Input: part model. Units: mm. Frame: model coordinates. Face numbers are marked on the shaded views. A direction names the side the tool comes from. Coordinates: 2 decimals unless noted, no trailing zeros. Write each loop counter-clockwise with the first axis right and the second up, starting at its lowest first coordinate (ties: lowest second). Pieces come first, ordered by that corner, then holes.
1) Section query A-A (y = 8). Output: boundary loops of the cut face in (x, z), then the cut area to 3 significant figures.
2) Section query B-B (z = 3.75). Output: boundary loops of the cut face in (x, y), then the cut area to 3 significant figures.
3) Pin query (flat end, axial travel): pin 1 Ø1.5 at (x, z) = (-2.5, 3.5) entering from -Y; pin 2 Ø0.7 at (x, y) = (5, 0) entering from +Z; pin 3 Ø3.5 at (x, z) = (-3.5, 2.5) entering from +Y; pin 4 Ø8 at (x, y) = (-16.5, 3) entering from -Z. Return the tip coordinate at first contact, or that it passes through.
4) Section query C-C (y = 0). Output: boundary loops of the cut face in (x, z), then the cut area to 3 significant figures.
5) Set-up query: the marked faces 1, 2 and 3. Return all of +Z, -Z, +X, -X, +Y, -Y with unobstructed straight access to the full face (end or side cutting, diameter ignored); none if empty.
6) Line query: L1, parallel to X at y = 4.75, z = -1; L2, parallel to Y at x = -33, z = 3.75; L3, parallel to Z at x = -10, y = -0.25. Output: solid intervals per line, ascending.
7) Section query D-D (x = -31). Output: boundary loops of the cut face in (y, z), then the cut area to 3 significant figures.
from build123d import *

# Parameters (mm, degrees)
SKETCH1_W           = 70
SKETCH1_H           = 5
SKETCH1_W_2         = 67
SKETCH1_H_2         = 1.4
BOSS_EXTRUDE1_DEPTH = 5
SKETCH2_W           = 70
SKETCH2_H           = 5
BOSS_EXTRUDE2_DEPTH = 2
BOSS_EXTRUDE3_DEPTH = 2.5
BOSS_EXTRUDE4_DEPTH = 2.5


with BuildPart() as part:
    # Sketch1 → Boss-Extrude1 (new body)
    with BuildSketch(Plane.XY):
        Rectangle(SKETCH1_W, SKETCH1_H)
        Rectangle(SKETCH1_W_2, SKETCH1_H_2, mode=Mode.SUBTRACT)
    extrude(amount=BOSS_EXTRUDE1_DEPTH)

    # Sketch2 → Boss-Extrude2 (add)
    with BuildSketch(Plane(origin=(0, 0, 0), x_dir=(-1, 0, 0), z_dir=(0, 0, -1))):
        Rectangle(SKETCH2_W, SKETCH2_H)
    extrude(amount=BOSS_EXTRUDE2_DEPTH)

    # Sketch3 → Boss-Extrude3 (add)
    with BuildSketch(Plane(origin=(35, 0, 0), x_dir=(0, 0, -1), z_dir=(1, 0, 0))):
        Polygon((-5, 2.5), (2, 15), (2, -15), (-5, -2.5), align=None)
    extrude(amount=BOSS_EXTRUDE3_DEPTH)

    # Sketch4 → Boss-Extrude4 (add)
    with BuildSketch(Plane.ZY.offset(35)):
        Polygon((5, 2.5), (-2, 15), (-2, -15), (5, -2.5), align=None)
    extrude(amount=BOSS_EXTRUDE4_DEPTH)


solid = part.part
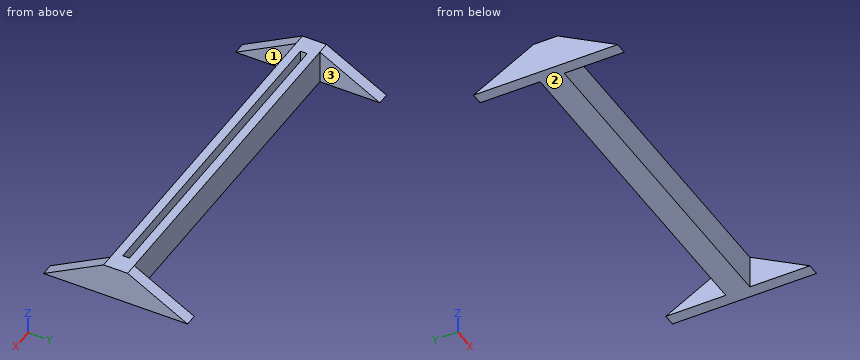
Answer:
1. outline: (-37.5, -2) - (-35, -2) - (-35, 1.92) - (-37.5, 1.92) - close; (35, -2) - (37.5, -2) - (37.5, 1.92) - (35, 1.92) - close
1. area: 19.6 mm2
2. outline: (-37.5, -4.73) - (-35, -4.73) - (-35, -2.5) - (35, -2.5) - (35, -4.73) - (37.5, -4.73) - (37.5, 4.73) - (35, 4.73) - (35, 2.5) - (-35, 2.5) - (-35, 4.73) - (-37.5, 4.73) - close; hole (-33.5, -0.7) - (33.5, -0.7) - (33.5, 0.7) - (-33.5, 0.7) - close
2. area: 304 mm2
3. pin 1: stops at y = -2.5
3. pin 2: stops at z = 0
3. pin 3: stops at y = 2.5
3. pin 4: stops at z = -2
4. outline: (-37.5, -2) - (37.5, -2) - (37.5, 5) - (33.5, 5) - (33.5, 0) - (-33.5, 0) - (-33.5, 5) - (-37.5, 5) - close
4. area: 190 mm2
5. face 1: +Z, -Z, -Y
5. face 2: -Z, +X, -X, +Y, -Y
5. face 3: +Z, -Z, +Y
6. L1: x = -37.5 to -35, 35 to 37.5
6. L2: y = -2.5 to -0.7, 0.7 to 2.5
6. L3: z = -2 to 0
7. outline: (-2.5, -2) - (2.5, -2) - (2.5, 5) - (0.7, 5) - (0.7, 0) - (-0.7, 0) - (-0.7, 5) - (-2.5, 5) - close
7. area: 28.0 mm2
